Check sheet for the drawn part. Datum: minimum x, y, z corner. Units: mm. A direction names the side the tool comes from. Round coordinates to 2 decimals unless told otherwise and drop trailing zeros. Order: outer loops, then holes, each group sorted by start corner. A loop starts at its lowest first (then second) coordinate and runs counter-clockwise, first axis right, second up. Notation, with made-up numbers: (55, 14.5) -> (110, 14.5) arc R8 cw to (110, 19.5) -> close; hole circle Ø4 at (84.5, -11). An arc over 180 degrees is marked (long way). Write item = value, one per line. Start each with the question number.
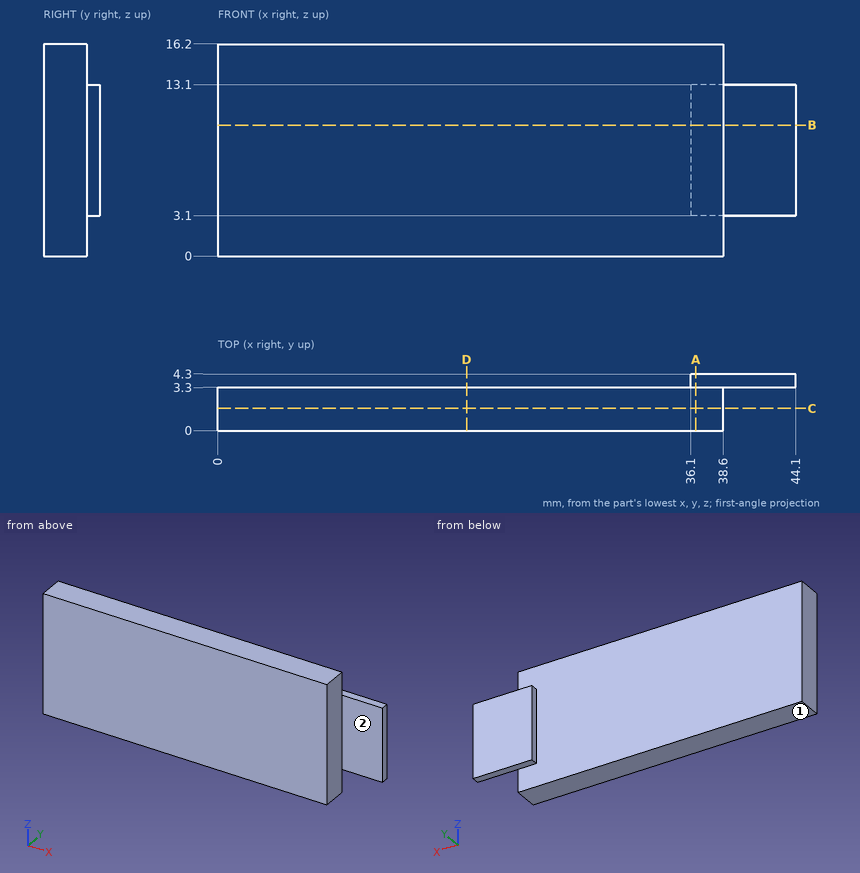
(1) Cross-section at D-D (x = 19). Enter the section's corners in (y, z), and give its area (3 significant figures).
(2) Cross-section at A-A (x = 36.5). Enter the section's corners in (y, z).
(3) Cross-section at B-B (z = 10). Enter the section's corners in (x, y), and give its area (3 significant figures).
(4) Set-up check for the marked faces 1 and 2: record each of +Z, -Z, +X, -X, +Y, -Y from which the full face is reachable in a straight line by a thin tool's end or side.
(5) Depth check by flat-ended pin: pin 1 (6 mm diameter, centred on x = 42.5, z = 6, fed in from -Y); pin 2 (2 mm diameter, centred on y = 1, z = 5, fed in from +X); pin 3 (8 mm diameter, centred on x = 23.5, z = 5, fed in from +Y). Enter the tip coordinate at first touch or a pass-through.
(6) Cross-section at C-C (y = 1.7). Enter the section's corners in (x, z), and give its area (3 significant figures).
(7) Scan lines: line 1 along Y through (x, z) = (8, 6); line 2 along X through (y, z) = (0.55, 12.5); line 3 along X through (y, z) = (3.8, 9.5). Record each from-to range of solid material in increasing order. Write a range as from..to.
Outcome:
q1.outline = (0, 0) -> (3.3, 0) -> (3.3, 16.2) -> (0, 16.2) -> close
q1.area = 53.5 mm^2
q2.outline = (0, 0) -> (3.3, 0) -> (3.3, 3.1) -> (4.3, 3.1) -> (4.3, 13.1) -> (3.3, 13.1) -> (3.3, 16.2) -> (0, 16.2) -> close
q3.outline = (0, 0) -> (38.6, 0) -> (38.6, 3.3) -> (44.1, 3.3) -> (44.1, 4.3) -> (36.1, 4.3) -> (36.1, 3.3) -> (0, 3.3) -> close
q3.area = 135 mm^2
q4.face_1 = -Z, +X, -X, +Y, -Y
q4.face_2 = +Z, -Z, +X, -Y
q5.pin_1 = 3.3
q5.pin_2 = 38.6
q5.pin_3 = 3.3
q6.outline = (0, 0) -> (38.6, 0) -> (38.6, 16.2) -> (0, 16.2) -> close
q6.area = 625 mm^2
q7.line_1 = 0..3.3
q7.line_2 = 0..38.6
q7.line_3 = 36.1..44.1
